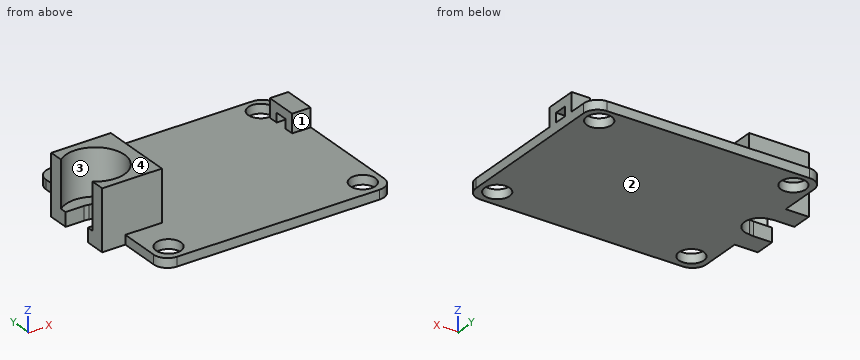
from build123d import *

# Parameters (mm, degrees)
CROQUIS1_W              = 49.8
CROQUIS1_H              = 39.8
CROQUIS1_R              = 2.7
SALIENTE_EXTRUIR1_DEPTH = 6
CORTAR_EXTRUIR1_DEPTH   = 4
REDONDEO1_R             = 3
SALIENTE_EXTRUIR3_DEPTH = 3
CROQUIS5_R              = 6.35
CORTAR_EXTRUIR2_DEPTH   = 3
SALIENTE_EXTRUIR4_DEPTH = 10
SALIENTE_EXTRUIR5_DEPTH = 2
CORTAR_EXTRUIR3_START   = -3
CORTAR_EXTRUIR3_DEPTH   = 3
CORTAR_EXTRUIR4_DEPTH   = 4
CROQUIS10_W             = 4
CROQUIS10_H             = 7
SALIENTE_EXTRUIR6_DEPTH = 4
CORTAR_EXTRUIR5_START   = -4
CORTAR_EXTRUIR5_DEPTH   = 4


with BuildPart() as part:
    # Croquis1 → Saliente-Extruir1 (new body)
    with BuildSketch(Plane.XY):
        with Locations((-31.963412372, -3.757931034)):
            Rectangle(CROQUIS1_W, CROQUIS1_H)
        with Locations((-52.963412372, 12.342068966)):
            Circle(CROQUIS1_R, mode=Mode.SUBTRACT)
        with Locations((-10.963412372, 12.342068966)):
            Circle(CROQUIS1_R, mode=Mode.SUBTRACT)
        with Locations((-10.963412372, -19.657931034)):
            Circle(CROQUIS1_R, mode=Mode.SUBTRACT)
        with Locations((-52.963412372, -19.657931034)):
            Circle(CROQUIS1_R, mode=Mode.SUBTRACT)
    extrude(amount=SALIENTE_EXTRUIR1_DEPTH)

    # Croquis2 → Cortar-Extruir1 (cut)
    with BuildSketch(Plane.XY.offset(6)):
        with BuildLine():
            Line((-49.963412372, -16.757931034), (-13.963412372, -16.757931034))
            ThreePointArc((-13.963412372, -16.757931034), (-12.54919881, -16.172144597), (-11.963412372, -14.757931034))
            Line((-11.963412372, -14.757931034), (-11.963412372, 7.242068966))
            ThreePointArc((-11.963412372, 7.242068966), (-12.54919881, 8.656282528), (-13.963412372, 9.242068966))
            Line((-13.963412372, 9.242068966), (-49.963412372, 9.242068966))
            ThreePointArc((-49.963412372, 9.242068966), (-51.377625934, 8.656282528), (-51.963412372, 7.242068966))
            Line((-51.963412372, 7.242068966), (-51.963412372, -14.757931034))
            ThreePointArc((-51.963412372, -14.757931034), (-51.377625934, -16.172144597), (-49.963412372, -16.757931034))
        make_face()
    extrude(amount=-CORTAR_EXTRUIR1_DEPTH, mode=Mode.SUBTRACT)

    # Redondeo1
    redondeo1_edges = [part.edges().sort_by_distance(p)[0] for p in [
        (-56.863412372, 16.142068966, 3),
        (-7.063412372, 16.142068966, 3),
        (-7.063412372, -23.657931034, 3),
        (-56.863412372, -23.657931034, 3),
    ]]
    fillet(redondeo1_edges, radius=REDONDEO1_R)

    # Croquis4 → Saliente-Extruir3 (add)
    with BuildSketch(Plane(origin=(0, 0, 0), x_dir=(-1, 0, 0), z_dir=(0, 0, -1))):
        with BuildLine():
            Line((56.863412372, 4.242068966), (61.863412372, 4.242068966))
            Line((61.863412372, 4.242068966), (61.863412372, -0.257931034))
            Line((61.863412372, -0.257931034), (57.863412372, -0.257931034))
            ThreePointArc((57.863412372, -0.257931034), (57.358118834, -0.294597605), (56.863412372, -0.403829068))
            Line((56.863412372, -0.403829068), (56.863412372, 4.242068966))
        make_face()
        with BuildLine():
            Line((61.863412372, -11.757931034), (56.863412372, -11.757931034))
            Line((56.863412372, -11.757931034), (56.863412372, -7.112033001))
            ThreePointArc((56.863412372, -7.112033001), (57.358118834, -7.221264464), (57.863412372, -7.257931034))
            Line((57.863412372, -7.257931034), (61.863412372, -7.257931034))
            Line((61.863412372, -7.257931034), (61.863412372, -11.757931034))
        make_face()
    extrude(amount=-SALIENTE_EXTRUIR3_DEPTH)

    # Croquis5 → Cortar-Extruir2 (cut)
    with BuildSketch(Plane.XY.offset(3)):
        with Locations((-57.863412372, -3.757931034)):
            Circle(CROQUIS5_R)
    extrude(amount=CORTAR_EXTRUIR2_DEPTH, mode=Mode.SUBTRACT)

    # Croquis6 → Saliente-Extruir4 (add)
    with BuildSketch(Plane.XY.offset(3)):
        with BuildLine():
            Line((-61.863412372, 4.242068966), (-51.963412372, 4.242068966))
            Line((-51.963412372, 4.242068966), (-48.963412372, 4.242068966))
            Line((-48.963412372, 4.242068966), (-48.963412372, -11.757931034))
            Line((-48.963412372, -11.757931034), (-51.963412372, -11.757931034))
            Line((-51.963412372, -11.757931034), (-61.863412372, -11.757931034))
            Line((-61.863412372, -11.757931034), (-61.863412372, -8.689715701))
            ThreePointArc((-61.863412372, -8.689715701), (-51.513412372, -3.757931034), (-61.863412372, 1.173853632))
            Line((-61.863412372, 1.173853632), (-61.863412372, 4.242068966))
        make_face()
    extrude(amount=SALIENTE_EXTRUIR4_DEPTH)

    # Croquis7 → Saliente-Extruir5 (add)
    with BuildSketch(Plane.XY.offset(2)):
        Polygon((-51.963412372, -3.757931034), (-51.963412372, 4.242068966), (-48.963412372, 4.242068966), (-48.963412372, -11.757931034), (-51.963412372, -11.757931034), align=None)
    extrude(amount=SALIENTE_EXTRUIR5_DEPTH)

    # Croquis8 → Cortar-Extruir3 (cut)
    with BuildSketch(Plane.XY.offset(3).offset(CORTAR_EXTRUIR3_START)):
        with BuildLine():
            Line((-56.863412372, -0.403829068), (-56.863412372, -7.112033001))
            ThreePointArc((-56.863412372, -7.112033001), (-53.509310406, -3.757931034), (-56.863412372, -0.403829068))
        make_face()
    extrude(amount=CORTAR_EXTRUIR3_DEPTH, mode=Mode.SUBTRACT)

    # Croquis9 → Cortar-Extruir4 (cut)
    with BuildSketch(Plane.XY.offset(6)):
        Polygon((-56.863412372, -11.757931034), (-56.863412372, -27.492217147), (-1.817084798, -27.492217147), (-1.817084798, 22.861833321), (-56.863412372, 22.861833321), (-56.863412372, 4.242068966), (-47.172737702, 4.242068966), (-47.172737702, -11.757931034), align=None)
    extrude(amount=-CORTAR_EXTRUIR4_DEPTH, mode=Mode.SUBTRACT)

    # Croquis10 → Saliente-Extruir6 (add)
    with BuildSketch(Plane.XY.offset(2)):
        with Locations((-9.063412372, 5.842068966)):
            Rectangle(CROQUIS10_W, CROQUIS10_H)
    extrude(amount=SALIENTE_EXTRUIR6_DEPTH)

    # Croquis11 → Cortar-Extruir5 (cut)
    with BuildSketch(Plane(origin=(-7.063412372, 0, 0), x_dir=(0, 0, -1), z_dir=(1, 0, 0)).offset(CORTAR_EXTRUIR5_START)):
        Polygon((-2, 5.842068966), (-2, 7.242068966), (-4, 7.242068966), (-4, 4.442068966), (-2, 4.442068966), align=None)
    extrude(amount=CORTAR_EXTRUIR5_DEPTH, mode=Mode.SUBTRACT)


solid = part.part
Design review of the part built by this model. Coordinates are the model's own, in mm. Face numbers are marked on the shaded views. A direction names the side the tool comes from. Coordinates: 2 decimals unless noted, no trailing zeros. Order: outer loops, then holes, each group sorted by start corner. A loop starts at its lowest first (then second) coordinate and runs counter-clockwise, first axis right, second up. Notation, with made-up numbers: (12.5, 15.25) - (35.5, 15.25) arc R11 ccw to (35.5, 28.25) - close; hole circle Ø5 at (-40, 55.5). An arc over 180 degrees is marked (long way). Put each result on its own line as item: value.
1) Take a section at B-B, the plane x = -55. Give the boundary of the cut face in (y, z), and give its area (3 significant figures).
Response values:
outline: (-23.43, 0) - (-21.43, 0) - (-21.43, 2) - (-23.43, 2) - close; (-17.89, 0) - (-6.55, 0) - (-6.55, 3) - (-9.43, 3) - (-9.43, 13) - (-11.76, 13) - (-11.76, 2) - (-17.89, 2) - close; (-0.97, 0) - (10.57, 0) - (10.57, 2) - (4.24, 2) - (4.24, 13) - (1.91, 13) - (1.91, 3) - (-0.97, 3) - close; (14.11, 0) - (15.92, 0) - (15.92, 2) - (14.11, 2) - close
area: 110 mm²
2) Take a section at D-D, the plane y = -4.5. Give the boundary of the cut face in (x, z), and give its area (3 significant figures).
Response values:
outline: (-53.59, 0) - (-7.06, 0) - (-7.06, 2) - (-48.96, 2) - (-48.96, 13) - (-51.56, 13) - (-51.56, 4) - (-51.96, 4) - (-51.96, 3) - (-53.59, 3) - close
area: 124 mm²
3) Wall thickness on L1, parallel to X at y = 4, z = 5.5; L2, parallel to Y at x = -51.5, z = 1.25; L3, parallel to Y at x = -59, z = 1.5: over which ranges is each line inside the solid? List them lowest first. Write a range as from..to.
Response values:
L1: x = -61.86..-48.96, -11.06..-7.06
L2: y = -23.66..-21.93, -17.39..10.07, 14.61..16.14
L3: y = -11.76..-7.26, -0.26..4.24
4) Insertion check: P1, Ø5, axis at x = -10.96, y = 12.34, coming from the +Z side; P2, Ø0.6, axis at y = -14, z = 0.5, coming from the -X side; P3, Ø1.2, axis at x = -9.5, z = 4.5, coming from the -Y side; P4, Ø1.2, axis at x = -9.5, y = 5, coming from the +Z side. Each pin has a flat end and moves straight along its axis. Give the tip position at first contact, or say it passes through.
Response values:
P1: passes through
P2: stops at x = -56.86
P3: stops at y = 2.34
P4: stops at z = 6
5) The part is to be moulded in two halves that separate along X. For the marked faces 3 and 4, say which applies: released by +X, released by -X, zero draft, split by the parting line, or undercut.
Response values:
face 3: undercut
face 4: zero draft
6) Tool access review of the marked faces 1 and 2: name each direction out of +Z, -Z, +X, -X, +Y, -Y from which nothing blocks a thin tool from reaching the whole face with its end or side.
Response values:
face 1: +Z, +X, -Y
face 2: -Z, +X, -X, +Y, -Y
7) Take a section at C-C, the plane z = 1.25. Give the boundary of the cut face in (x, y), and give its area (3 significant figures).
Response values:
outline: (-61.86, -11.76) - (-56.86, -11.76) - (-56.86, -20.66) arc R3 ccw to (-53.86, -23.66) - (-10.06, -23.66) arc R3 ccw to (-7.06, -20.66) - (-7.06, 13.14) arc R3 ccw to (-10.06, 16.14) - (-53.86, 16.14) arc R3 ccw to (-56.86, 13.14) - (-56.86, 4.24) - (-61.86, 4.24) - (-61.86, -0.26) - (-57.86, -0.26) arc R3.5 cw to (-56.86, -0.4) arc R3.35 cw to (-56.86, -7.11) arc R3.5 cw to (-57.86, -7.26) - (-61.86, -7.26) - close; hole circle Ø5.4 at (-52.96, -19.66); hole circle Ø5.4 at (-52.96, 12.34); hole circle Ø5.4 at (-10.96, -19.66); hole circle Ø5.4 at (-10.96, 12.34)
area: 1,910 mm²
8) Take a section at A-A, the plane y = 11. Give the boundary of the cut face in (x, z).
Response values:
outline: (-56.86, 0) - (-55.31, 0) - (-55.31, 2) - (-56.86, 2) - close; (-50.62, 0) - (-13.31, 0) - (-13.31, 2) - (-50.62, 2) - close; (-8.62, 0) - (-7.06, 0) - (-7.06, 2) - (-8.62, 2) - close
